The model under review builds one solid part; all positions refer to its coordinate system, in mm. A direction names the side the tool comes from. Coordinates: 2 decimals unless noted, no trailing zeros. Write each loop counter-clockwise with the first axis right and the second up, starting at its lowest first coordinate (ties: lowest second). Pieces come first, ordered by that corner, then holes.
1) Machinability: for faces 1 (the flat face through (-1, -30.668, 13)), 2 (the cylindrical face through (-13.37, 0.59, 30.55)), which of the approach directions +Z, -Z, +X, -X, +Y, -Y give a long, thin tool a straight path to every point of the face, cutting with its end or side? Answer none if there is none.
2) Add section A-A, the plane y = 0. State the section outline as (x, z) points.
3) Add section C-C, the plane y = -25. State the section outline as (x, z) points, then the cut area to 3 significant figures.
4) For line 1 (Z direction, x = -15, y = 10); line 2 (Z direction, x = 6.5, y = -4); line 3 (X direction, y = -11, z = 27.5), list the stretches that pass through material, from the lowest coordinate up.
5) Add section D-D, the plane x = 16. State the section outline as (y, z) points, then the cut area to 3 significant figures.
6) Add section B-B, the plane x = -1. State the section outline as (y, z) points, then the cut area to 3 significant figures.
7) For P1, Ø10, axis at x = -10.5, z = 30, coming from the +Y side; P2, Ø12, axis at x = -23.5, y = 14, coming from the +Z side; P3, Ø2, axis at y = 12, z = 27.5, coming from the +X side, all flat-tipped, find the tip position at first contact; note any pin that passes through.
from build123d import *

# Parameters (mm, degrees)
F0_W     = 82.296788
F0_H     = 61.336212
F1_DEPTH = 25.4
F2_R     = 13.383079
F3_DEPTH = 14.986
F5_DEPTH = 25.4


with BuildPart() as f1:
    # F0 (on Top) → F1 (new body)
    with BuildSketch(Plane.XY):
        Rectangle(F0_W, F0_H)
    extrude(amount=F1_DEPTH)

    # F2 (on face) → F3 (join)
    with BuildSketch(Plane.XY.offset(25.4)):
        Circle(F2_R)
    extrude(amount=F3_DEPTH)

    # F4 (on Front) → F5 (cut, symmetric)
    with BuildSketch(Plane.XZ):
        Polygon((18.06845, 41.92983), (-21.930402, 41.92983), (18.06845, 26.757853), align=None)
    extrude(amount=F5_DEPTH, both=True, mode=Mode.SUBTRACT)


solid = f1.part
Geometry results:
1. face 1: +Z, -Z, +X, -X, -Y
1. face 2: +Z
2. outline: (-41.15, 0) - (41.15, 0) - (41.15, 25.4) - (13.38, 25.4) - (13.38, 28.54) - (-13.38, 38.69) - (-13.38, 25.4) - (-41.15, 25.4) - close
3. outline: (-41.15, 0) - (41.15, 0) - (41.15, 25.4) - (-41.15, 25.4) - close
3. area: 2,090 mm2
4. line 1: z = 0 to 25.4
4. line 2: z = 0 to 31.15
4. line 3: x = -7.62 to 7.62
5. outline: (-30.67, 0) - (30.67, 0) - (30.67, 25.4) - (-30.67, 25.4) - close
5. area: 1,560 mm2
6. outline: (-30.67, 0) - (30.67, 0) - (30.67, 25.4) - (13.35, 25.4) - (13.35, 33.99) - (-13.35, 33.99) - (-13.35, 25.4) - (-30.67, 25.4) - close
6. area: 1,790 mm2
7. P1: stops at y = 30.67
7. P2: stops at z = 25.4
7. P3: stops at x = 7.62
